from build123d import *

# Parameters (mm, degrees)
SKETCH1_R   = 4.826
SKETCH1_R_2 = 4.191


with BuildPart() as part:
    # Sweep1: sweep along a curve in space
    with BuildLine() as sweep1_path:
        Line((0, 0, 0), (0, 0, 44.45))
        ThreePointArc((0, 0, 44.45), (5.579615818, 0, 57.920384182), (19.05, 0, 63.5))
        Line((19.05, 0, 63.5), (228.6, 0, 63.5))
    # Sketch1 → Sweep1 (sweep)
    with BuildSketch(Plane.XY):
        Circle(SKETCH1_R)
        Circle(SKETCH1_R_2, mode=Mode.SUBTRACT)
    sweep(path=sweep1_path.line)


solid = part.part
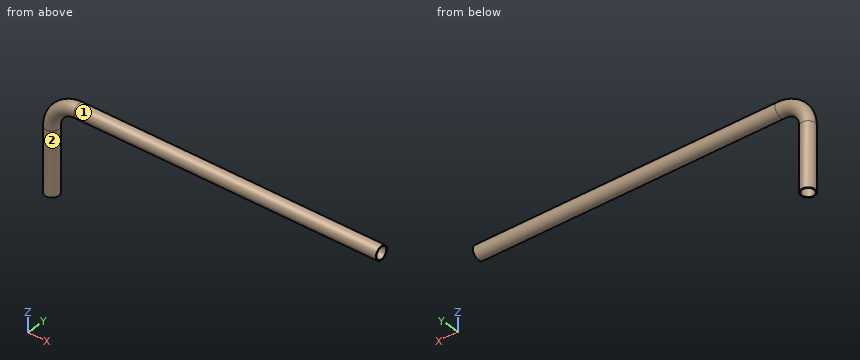
Work out the finished part from the listing and answer in its coordinate system (mm). Face numbers are marked on the shaded views. A direction names the side the tool comes from. Round coordinates to 2 decimals unless told otherwise and drop trailing zeros. Write each loop counter-clockwise with the first axis right and the second up, starting at its lowest first coordinate (ties: lowest second). Pieces come first, ordered by that corner, then holes.
1) A cutting plane is placed at A-A (y = 0). Give the vertices of the cut face in (x, z).
2) Straight lines are drawn through the part: line 1 (Y direction, x = 172, z = 63.5); line 2 (Z direction, x = 49.5, y = -0.5); line 3 (X direction, y = 3, z = 26.5). For each, find the intervals that lie inside material, in ascending order.
3) Given pin 1 Ø1.5 at (x, y) = (199.5, -1) entering from +Z; pin 2 Ø1.5 at (x, y) = (52.5, -2) entering from +Z; pin 3 Ø5 at (y, z) = (3.5, 31) entering from +X, each flat-ended and moving along its own axis, determine where each tip first touches the part or whether it passes through.
4) A tool of negligible diameter and unlimited length cuts with its end or side. For the marked faces 1 and 2, from which of +Z, -Z, +X, -X, +Y, -Y can it reach the whole face along a straight path? Write none if from no direction.
5) A cutting plane is placed at C-C (x = 163). Give the vertices of the cut face in (y, z).
6) A cutting plane is placed at B-B (z = 16). Give the vertices of the cut face in (x, y).
Completed:
1. outline: (-4.83, 0) - (-4.19, 0) - (-4.19, 44.45) arc R23.24 cw to (19.05, 67.69) - (228.6, 67.69) - (228.6, 68.33) - (19.05, 68.33) arc R23.88 ccw to (-4.83, 44.45) - close; (4.19, 0) - (4.83, 0) - (4.83, 44.45) arc R14.22 cw to (19.05, 58.67) - (228.6, 58.67) - (228.6, 59.31) - (19.05, 59.31) arc R14.86 ccw to (4.19, 44.45) - close
2. line 1: y = -4.83 to -4.19, 4.19 to 4.83
2. line 2: z = 58.7 to 59.34, 67.66 to 68.3
2. line 3: x = -3.78 to -2.93, 2.93 to 3.78
3. pin 1: stops at z = 68.32
3. pin 2: stops at z = 68.16
3. pin 3: stops at x = 4.72
4. face 1: +X
4. face 2: -Z
5. outline: circle Ø9.65 at (0, 63.5); hole circle Ø8.38 at (0, 63.5)
6. outline: circle Ø9.65 at (0, 0); hole circle Ø8.38 at (0, 0)
